```python
from build123d import *

# Parameters (mm, degrees)
F0_W     = 101.6
F0_H     = 25.4
F0_R     = 6.35
F0_W_2   = 12.7
F0_H_2   = 12.7
F1_DEPTH = 0.3


with BuildPart() as f1:
    # F0 (on Top) → F1 (new body)
    with BuildSketch(Plane.XY):
        with Locations((50.8, 12.7)):
            Rectangle(F0_W, F0_H)
        Polygon((9.469252, 18.295827), (15.818924, 18.360389), (19.049672, 12.893693), (15.930748, 7.362435), (9.581076, 7.297873), (6.350328, 12.764569), align=None, mode=Mode.SUBTRACT)
        with Locations((50.8, 13.216523)):
            Circle(F0_R, mode=Mode.SUBTRACT)
        with Locations((88.9, 13.603915)):
            Rectangle(F0_W_2, F0_H_2, mode=Mode.SUBTRACT)
    extrude(amount=F1_DEPTH)


solid = f1.part
```
For this review, take the finished solid that the model builds, in its own axes (mm). Coordinates: 2 decimals unless noted, no trailing zeros. Loops run counter-clockwise (first coordinate to the right, second up) from the corner with the lowest first, then second, coordinate; pieces in that order, holes last.
1. Add section A-A, the plane x = 50.8. Give the boundary of the cut face in (y, z), then the cut area to 3 significant figures.
2. Add section C-C, the plane z = 0.1. Give the boundary of the cut face in (x, y).
3. Insertion check: P1, Ø11.5, axis at x = 50.8, y = 13.22, coming from the +Z side; P2, Ø6, axis at x = 89.5, y = 22, coming from the -Z side. Each pin has a flat end and moves straight along its axis. Give the tip position at first contact, or say it passes through.
4. Mouldability with a two-part tool opening along X and no side actions: class faces 1 (the flat face through (39, 13, 0.3)), 2 (the cylindrical face through (49.42, 7.02, 0.15)) as +X half, -X half, draft (parallel to the pull), parting line (faces both ways), or undercut.
5. For line 1 (X direction, y = 9.5, z = 0.15); line 2 (X direction, y = 11.5, z = 0.15); line 3 (Y direction, x = 50.8, z = 0.15), list the stretches that pass through material, from the lowest coordinate up.
6. Add section B-B, the plane y = 10. Give the boundary of the cut face in (x, z).
Result:
1. outline: (0, 0) - (6.87, 0) - (6.87, 0.3) - (0, 0.3) - close; (19.57, 0) - (25.4, 0) - (25.4, 0.3) - (19.57, 0.3) - close
1. area: 3.81 mm2
2. outline: (0, 0) - (101.6, 0) - (101.6, 25.4) - (0, 25.4) - close; hole (6.35, 12.76) - (9.58, 7.3) - (15.93, 7.36) - (19.05, 12.89) - (15.82, 18.36) - (9.47, 18.3) - close; hole circle Ø12.7 at (50.8, 13.22); hole (82.55, 7.25) - (95.25, 7.25) - (95.25, 19.95) - (82.55, 19.95) - close
3. P1: passes through
3. P2: stops at z = 0
4. face 1: draft
4. face 2: undercut
5. line 1: x = 0 to 8.28, 17.14 to 45.65, 55.95 to 82.55, 95.25 to 101.6
5. line 2: x = 0 to 7.1, 18.26 to 44.69, 56.91 to 82.55, 95.25 to 101.6
5. line 3: y = 0 to 6.87, 19.57 to 25.4
6. outline: (0, 0) - (7.98, 0) - (7.98, 0.3) - (0, 0.3) - close; (17.42, 0) - (45.32, 0) - (45.32, 0.3) - (17.42, 0.3) - close; (56.28, 0) - (82.55, 0) - (82.55, 0.3) - (56.28, 0.3) - close; (95.25, 0) - (101.6, 0) - (101.6, 0.3) - (95.25, 0.3) - close
